Geometry check sheet. Reference: the model listing, model coordinates, mm. A direction names the side the tool comes from. Give positions to 0.01 mm unless a question says otherwise; leave off trailing zeros. Write each loop counter-clockwise with the first axis right and the second up, starting at its lowest first coordinate (ties: lowest second). Pieces come first, ordered by that corner, then holes. Notation, with made-up numbers: (-23.5, 48.25) -> (30.5, 48.25) arc R16 ccw to (30.5, 56.25) -> close; hole circle Ø2 at (13.25, -39.5). An arc over 180 degrees is marked (long way). Use a Markdown table: item, result. Add a question column.
Autodesk Inventor part; units mm, degrees
ref_plane "Work Plane1" through (0, 0, 0) normal (0, 0, 1) x (1, 0, 0)
ref_plane "YZ Plane" through (0, 0, 0) normal (1, 0, 0) x (0, 1, 0)
ref_plane "XZ Plane" through (0, 0, 0) normal (0, 1, 0) x (-1, 0, 0)
sketch "Sketch1" plane through (0, 0, 0) normal (0, 0, 1) x (1, 0, 0)
  line L0 (-35, 30) -> (35, 30)
  line L1 (35, 30) -> (35, -30)
  line L2 (35, -30) -> (-35, -30)
  line L3 (-35, -30) -> (-35, 30)
  point P0 (0, 0)
  point P1 (0, 30)
  point P2 (-35, 0)
  dimension "d0" = 70
  dimension "d1" = 60
extrude "Extrusion1" add sketch "Sketch1" along normal mid plane 103.5
sketch "Sketch2" plane through (-35, 30, 51.75) normal (0, 1, 0) x (1, 0, 0)
  line L0 (0, 103.5) -> (70, 103.5)
  line L1 (5, 98.5) -> (65, 98.5)
  line L2 (65, 98.5) -> (65, 5)
  line L3 (65, 5) -> (5, 5)
  line L4 (5, 5) -> (5, 98.5)
  point P0 (35, 51.75)
  point P1 (5, 51.75)
  point P2 (35, 98.5)
  point P3 (35, 103.5)
  dimension "d4" = 93.5
  dimension "d5" = 60
extrude "Extrusion2" cut sketch "Sketch2" against normal blind 55
fillet "Fillet2" radius 3 8 edges at (35, 0, 51.75) (35, 0, -51.75) (-35, 0, 51.75) (-35, 0, -51.75) (35, -30, 0) (0, -30, 51.75) (-35, -30, 0) (0, -30, -51.75)
ref_plane "Work Plane1" through (0, 0, 0) normal (0, 0, 1) x (1, 0, 0)
sketch "Sketch3" plane through (0, 0, 0) normal (0, 0, 1) x (1, 0, 0)
  line L0 (-30, 30) -> (-30, -25)
  line L1 (-30, 25) -> (-32, 24)
  line L2 (-32, 24) -> (-32, 22)
  line L3 (-32, 30) -> (-32, -27)
  line L4 (-32, 22) -> (-30, 21)
  line L5 (-30, 21) -> (-30, 25)
  point P0 (0, 0)
  point P1 (-32, -25)
  dimension "d12" = 5
  dimension "d13" = 4
  dimension "d14" = 2
  dimension "d15" = 2
extrude "Extrusion3" cut sketch "Sketch3" along normal mid plane 93.5
mirror "Mirror1" about plane through (0, 0, 0) normal (1, 0, 0) of "Extrusion3"
sketch "Sketch8" plane through (35, -27, 48.75) normal (1, 0, 0) x (0, 0, -1)
  line L0 (97.5, 57) -> (0, 57)
  circle A0 centre (54.5, 30.5) radius 5.45
  line L1 (100.5, 0) -> (100.5, 57)
  line L2 (2, 2) -> (95.5, 2)
  point P0 (48.75, 27)
  dimension "d31" = 46
  dimension "d32" = 28.5
  dimension "d33" = 10.9
extrude "Extrusion7" add sketch "Sketch8" along normal blind 1
sketch "Sketch9" plane through (36, 3.5, -5.75) normal (1, 0, 0) x (0, 0, -1)
  circle A0 centre (0, 0) radius 5.45
  circle A1 centre (0, 0) radius 2.45
  point P0 (-5.75, -3.5)
  dimension "d36" = 4.9
extrude "Extrusion8" cut sketch "Sketch9" against normal up to surface (6 mm away) contours A1
chamfer "Chamfer1" distance 1 angle 45 3 edges at (36, 3.5, -3.3) (36, 3.5, -0.3) (30, 3.5, -3.3)
sketch "Sketch10" plane through (35, -27, 48.75) normal (1, 0, 0) x (0, 0, -1)
  line L0 (14.5, 26) -> (28.5, 26)
  line L1 (28.5, 26) -> (28.5, 37)
  line L2 (28.5, 37) -> (14.5, 37)
  line L3 (14.5, 37) -> (14.5, 26)
  line L4 (2, 48) -> (2, 2)
  line L5 (95.5, 2) -> (2, 2)
  point P0 (48.75, 27)
  dimension "d42" = 12.5
  dimension "d44" = 11
  dimension "d45" = 14
  dimension "d58" = 24
extrude "Extrusion9" cut sketch "Sketch10" against normal blind 2
sketch "Sketch11" plane through (33, -27, 48.75) normal (1, 0, 0) x (0, 0, -1)
  line L0 (17.5, 34) -> (25.5, 34)
  line L1 (25.5, 34) -> (25.5, 29)
  line L2 (25.5, 29) -> (17.5, 29)
  line L3 (17.5, 29) -> (17.5, 34)
  line L4 (14.5, 37) -> (28.5, 37)
  line L5 (14.5, 26) -> (14.5, 37)
  point P0 (48.75, 27)
  point P1 (17.5, 31.5)
  point P2 (14.5, 31.5)
  point P3 (21.5, 37)
  point P4 (21.5, 34)
  dimension "d48" = 5
  dimension "d49" = 8
extrude "Extrusion10" cut sketch "Sketch11" against normal up to surface (3 mm away)
chamfer "Chamfer2" distance 1 angle 45 4 edges at (35, 10, 27.25) (35, 4.5, 20.25) (35, 4.5, 34.25) (35, -1, 27.25)
properties part number "Part_A1"
1) Tool access check on faces 4 (the face through (33, 8, 27)), 5 (the face through (30, -2, -1)), 6 (the face through (-34.14, -29.1, 0.68)). Record the directions out of +Z, -Z, +X, -X, +Y, -Y that give a thin tool (end or side, any length) a straight path to the whole face; none if there is none.
2) Sectioned sample at C-C, the plane z = 38. Enter the section's corners in (x, y), and give its area (3 significant figures).
3) Sectioned sample at D-D, the plane x = 27. Enter the section's corners in (y, z).
4) Material ranges on probe 1 along X at (y, z) = (22, -9); probe 2 along Z at (x, y) = (-9, -23.5); probe 3 along X at (y, z) = (-8, -24.5), recorded low to high. Write a range as [from, to].
5) Sectioned sample at B-B, the plane y = -20. Enter the section's corners in (x, z).
6) Draft check along Z on faces 1 (the face through (-34.14, 1.9, 50.85)), 2 (the face through (34.1, 1.1, -50.89)), 3 (the face through (32, 4, 31.25)). Enter one of: +Z half, -Z half, draft (parallel to the pull), parting line (faces both ways), or undercut.
7) Gauge pin test, flat ends, axial feed: P1, Ø12, axis at x = -5, z = -19.5, coming from the +Y side; P2, Ø2, axis at y = 22.5, z = 13.5, coming from the +X side; P3, Ø3, axis at y = 3.5, z = -5.75, coming from the +X side. Record the tip position at first contact, or that the pin passes through.
Check values:
| question | item | result |
|---|---|---|
| 1 | face 4 | +X |
| 1 | face 5 | +Y |
| 1 | face 6 | +Z, -Z, -X, -Y |
| 2 | outline | (-35, -27) arc R3 ccw to (-32, -30) -> (32, -30) arc R3 ccw to (35, -27) -> (35, 30) -> (30, 30) -> (30, 25) -> (32, 24) -> (32, 22) -> (30, 21) -> (30, -25) -> (-30, -25) -> (-30, 21) -> (-32, 22) -> (-32, 24) -> (-30, 25) -> (-30, 30) -> (-35, 30) -> close |
| 2 | area | 884 mm² |
| 3 | outline | (-30, -48.75) arc R3 ccw to (-27, -51.75) -> (30, -51.75) -> (30, -46.75) -> (-25, -46.75) -> (-25, 46.75) -> (30, 46.75) -> (30, 51.75) -> (-27, 51.75) arc R3 ccw to (-30, 48.75) -> close |
| 4 | probe 1 | [-35, -32], [32, 35] |
| 4 | probe 2 | [-51.75, -46.75], [46.75, 51.75] |
| 4 | probe 3 | [-35, -30], [30, 35] |
| 5 | outline | (-35, -48.75) arc R3 ccw to (-32, -51.75) -> (32, -51.75) arc R3 ccw to (35, -48.75) -> (35, 48.75) arc R3 ccw to (32, 51.75) -> (-32, 51.75) arc R3 ccw to (-35, 48.75) -> close; hole (-30, -46.75) -> (30, -46.75) -> (30, 46.75) -> (-30, 46.75) -> close |
| 6 | face 1 | +Z half |
| 6 | face 2 | -Z half |
| 6 | face 3 | undercut |
| 7 | P1 | y = -25 |
| 7 | P2 | x = 35 |
| 7 | P3 | x = -30 |
